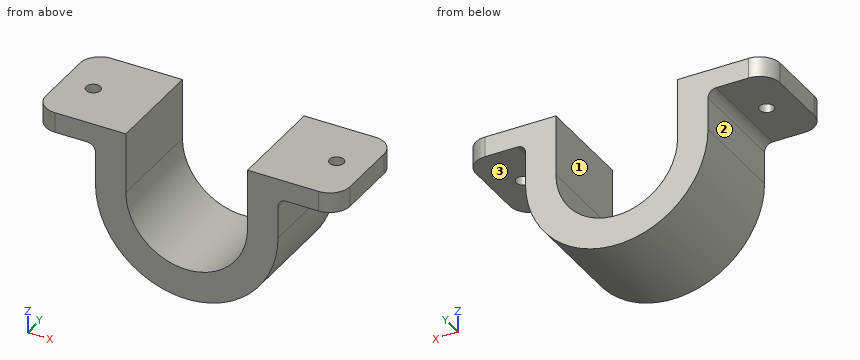
```python
from build123d import *

# Parameters (mm, degrees)
BOSS_EXTRUDE1_DEPTH = 25
SKETCH4_R           = 1.75
CUT_EXTRUDE1_DEPTH  = 6
FILLET1_R           = 5
FILLET2_R           = 2


with BuildPart() as part:
    # Sketch1 → Boss-Extrude1 (new body)
    with BuildSketch(Plane(origin=(0, 0, 0), x_dir=(1, 0, 0), z_dir=(0, 1, 0))):
        with BuildLine():
            Line((-7.5, 0), (-7.5, -10))
            Line((-7.5, -10), (-22.5, -10))
            Line((-22.5, -10), (-22.5, -15))
            Line((-22.5, -15), (0, -15))
            Line((0, -15), (0, 0))
            ThreePointArc((0, 0), (15, 15), (30, 0))
            Line((30, 0), (30, -15))
            Line((30, -15), (52.5, -15))
            Line((52.5, -15), (52.5, -10))
            Line((52.5, -10), (37.5, -10))
            Line((37.5, -10), (37.5, 0))
            ThreePointArc((37.5, 0), (15, 22.5), (-7.5, 0))
        make_face()
    extrude(amount=BOSS_EXTRUDE1_DEPTH)

    # Sketch4 → Cut-Extrude1 (cut, through all)
    with BuildSketch(Plane(origin=(0, 0, 10), x_dir=(-1, 0, 0), z_dir=(0, 0, -1))):
        with Locations((-45, 12.5)):
            Circle(SKETCH4_R)
        with Locations((15, 12.5)):
            Circle(SKETCH4_R)
    extrude(amount=-CUT_EXTRUDE1_DEPTH, mode=Mode.SUBTRACT)

    # Fillet1
    fillet1_edges = [part.edges().sort_by_distance(p)[0] for p in [
        (-22.5, 0, 12.5),
        (52.5, 0, 12.5),
        (52.5, 25, 12.5),
        (-22.5, 25, 12.5),
    ]]
    fillet(fillet1_edges, radius=FILLET1_R)

    # Fillet2
    fillet2_edges = [part.edges().sort_by_distance(p)[0] for p in [
        (-7.5, 12.5, 10),
        (37.5, 12.5, 10),
    ]]
    fillet(fillet2_edges, radius=FILLET2_R)


solid = part.part
```
Geometry: final body of the model. Coordinates: model frame, mm. Face numbers are marked on the shaded views. A direction names the side the tool comes from. Coordinates: 2 decimals unless noted, no trailing zeros. Order: outer loops, then holes, each group sorted by start corner. A loop starts at its lowest first (then second) coordinate and runs counter-clockwise, first axis right, second up. Notation, with made-up numbers: (59.5, 50) - (82.5, 50) arc R10 cw to (82.5, 54) - close; hole circle Ø2 at (89.5, 85). An arc over 180 degrees is marked (long way). Return JSON: item names as keys, results as strings. Group by question number.
1. Cut plane B-B (y = 12.5). Output: boundary loops of the cut face in (x, z), plus the area to 3 significant figures.
2. Material intervals for line 1 along Y through (x, z) = (45, 12.55); line 2 along X through (y, z) = (22.5, 2.5); line 3 along X through (y, z) = (7.25, 11.5), sorted ascending. Write a range as [from, to].
3. Cut plane A-A (z = 11). Output: boundary loops of the cut face in (x, y).
4. Pin query (flat end, axial travel): pin 1 (4 mm diameter, centred on x = -15.5, y = 14, fed in from -Z); pin 2 (5 mm diameter, centred on y = 5, z = -15, fed in from +X); pin 3 (9 mm diameter, centred on y = 12, z = 4, fed in from -X); pin 4 (1 mm diameter, centred on x = 9.5, z = -12, fed in from +Y). Return the tip coordinate at first contact, or that it passes through.
5. Cut plane C-C (z = 3). Output: boundary loops of the cut face in (x, y), plus the area to 3 significant figures.
6. Set-up query: the marked faces 1, 2 and 3. Return all of +Z, -Z, +X, -X, +Y, -Y with unobstructed straight access to the full face (end or side cutting, diameter ignored); none if empty.
7. Cut plane D-D (y = 7). Output: boundary loops of the cut face in (x, z), plus the area to 3 significant figures.
Resolved:
{
 "1": {"outline": "(-22.5, 10) - (-16.75, 10) - (-16.75, 15) - (-22.5, 15) - close; (-13.25, 10) - (-9.5, 10) arc R2 cw to (-7.5, 8) - (-7.5, 0) arc R22.5 ccw to (37.5, 0) - (37.5, 8) arc R2 cw to (39.5, 10) - (43.25, 10) - (43.25, 15) - (30, 15) - (30, 0) arc R15 cw to (0, 0) - (0, 15) - (-13.25, 15) - close; (46.75, 10) - (52.5, 10) - (52.5, 15) - (46.75, 15) - close", "area": "784 mm²"},
 "2": {"line 1": "y = [0, 10.75], [14.25, 25]", "line 2": "x = [-7.5, 0], [30, 37.5]", "line 3": "x = [-22.5, 0], [30, 52.5]"},
 "3": {"outline": "(-22.5, 5) arc R5 ccw to (-17.5, 0) - (0, 0) - (0, 25) - (-17.5, 25) arc R5 ccw to (-22.5, 20) - close; (30, 0) - (47.5, 0) arc R5 ccw to (52.5, 5) - (52.5, 20) arc R5 ccw to (47.5, 25) - (30, 25) - close; hole circle Ø3.5 at (-15, 12.5); hole circle Ø3.5 at (45, 12.5)"},
 "4": {"pin 1": "stops at z = 10", "pin 2": "stops at x = 33.71", "pin 3": "stops at x = -7.56", "pin 4": "passes through"},
 "5": {"outline": "(-7.5, 0) - (0, 0) - (0, 25) - (-7.5, 25) - close; (30, 0) - (37.5, 0) - (37.5, 25) - (30, 25) - close", "area": "375 mm²"},
 "6": {"face 1": "+Z, +Y, -Y", "face 2": "-Z, -X, +Y, -Y", "face 3": "-Z, +X, +Y, -Y"},
 "7": {"outline": "(-22.5, 10) - (-9.5, 10) arc R2 cw to (-7.5, 8) - (-7.5, 0) arc R22.5 ccw to (37.5, 0) - (37.5, 8) arc R2 cw to (39.5, 10) - (52.5, 10) - (52.5, 15) - (30, 15) - (30, 0) arc R15 cw to (0, 0) - (0, 15) - (-22.5, 15) - close", "area": "819 mm²"}
}
